from build123d import *

# Parameters (mm, degrees)
SKETCH1_W            = 61
SKETCH1_H            = 90
BOSS_EXTRUDE1_DEPTH  = 8
SKETCH4_W            = 57
SKETCH4_H            = 86
CUT_EXTRUDE1_DEPTH   = 6
SKETCH5_R            = 1.5
BOSS_EXTRUDE12_DEPTH = 2
CUT_EXTRUDE2_REACH   = 79.614
SKETCH6_R            = 3.5
SKETCH6_W            = 17
SKETCH6_H            = 6.5
SKETCH6_W_2          = 9.5
SKETCH6_H_2          = 4
CUT_EXTRUDE3_REACH   = 98.629
SKETCH8_W            = 17.9
SKETCH8_H            = 15.5
SKETCH8_W_2          = 15.1
SKETCH8_H_2          = 16


with BuildPart() as part:
    # Sketch1 → Boss-Extrude1 (new body)
    with BuildSketch(Plane(origin=(0, 0, 0), x_dir=(1, 0, 0), z_dir=(0, 1, 0))):
        Rectangle(SKETCH1_W, SKETCH1_H)
    extrude(amount=BOSS_EXTRUDE1_DEPTH)

    # Sketch4 → Cut-Extrude1 (cut)
    with BuildSketch(Plane(origin=(0, 2, 0), x_dir=(1, 0, 0), z_dir=(0, 1, 0))):
        Rectangle(SKETCH4_W, SKETCH4_H)
    extrude(amount=CUT_EXTRUDE1_DEPTH, mode=Mode.SUBTRACT)

    # Sketch5 → Boss-Extrude12 (add)
    # profile 1 of 4: a face of its own
    with BuildSketch(Plane(origin=(0, 2, 0), x_dir=(1, 0, 0), z_dir=(0, 1, 0))):
        with BuildLine():
            Line((25, -15), (28.5, -15))
            Line((28.5, -15), (28.5, -22))
            Line((28.5, -22), (25, -22))
            ThreePointArc((25, -22), (21.5, -18.5), (25, -15))
        make_face()
        with Locations(Location((25, -18.5, 0), (0, 0, 270))):
            Circle(SKETCH5_R, mode=Mode.SUBTRACT)
    # profile 2 of 4: a face of its own
    with BuildSketch(Plane(origin=(0, 2, 0), x_dir=(1, 0, 0), z_dir=(0, 1, 0))):
        with BuildLine():
            Line((31.5, 39.5), (31.5, 46))
            Line((31.5, 46), (25, 46))
            ThreePointArc((25, 46), (20.403805922, 34.903805922), (31.5, 39.5))
        make_face()
        with Locations(Location((25, 39.5, 0), (0, 0, 270))):
            Circle(SKETCH5_R, mode=Mode.SUBTRACT)
    # profile 3 of 4: a face of its own
    with BuildSketch(Plane(origin=(0, 2, 0), x_dir=(1, 0, 0), z_dir=(0, 1, 0))):
        with BuildLine():
            Line((-20.5, 39.5), (-20.5, 43))
            Line((-20.5, 43), (-28.5, 43))
            Line((-28.5, 43), (-28.5, 36))
            Line((-28.5, 36), (-24, 36))
            ThreePointArc((-24, 36), (-21.525126266, 37.025126266), (-20.5, 39.5))
        make_face()
        with Locations(Location((-24, 39.5, 0), (0, 0, 90))):
            Circle(SKETCH5_R, mode=Mode.SUBTRACT)
    # profile 4 of 4: a face of its own
    with BuildSketch(Plane(origin=(0, 2, 0), x_dir=(1, 0, 0), z_dir=(0, 1, 0))):
        with BuildLine():
            Line((-24, -15), (-28.506473373, -15))
            Line((-28.506473373, -15), (-28.5, -22))
            Line((-28.5, -22), (-24, -22))
            ThreePointArc((-24, -22), (-20.5, -18.5), (-24, -15))
        make_face()
        with Locations(Location((-24, -18.5, 0), (0, 0, 270))):
            Circle(SKETCH5_R, mode=Mode.SUBTRACT)
    extrude(amount=BOSS_EXTRUDE12_DEPTH)

    # Sketch6 → Cut-Extrude2 (cut, up to next)
    with BuildSketch(Plane.ZY.offset(30.5), mode=Mode.PRIVATE) as cut_extrude2_sk1:
        with Locations((10.5, 8.4)):
            Circle(SKETCH6_R)
    cut_extrude2_tool1 = extrude(cut_extrude2_sk1.sketch, amount=-CUT_EXTRUDE2_REACH, mode=Mode.PRIVATE) & part.part
    # Sketch6 → Cut-Extrude2 (cut, up to next)
    with BuildSketch(Plane.ZY.offset(30.5), mode=Mode.PRIVATE) as cut_extrude2_sk2:
        with Locations((-11, 8.15)):
            Rectangle(SKETCH6_W, SKETCH6_H)
    cut_extrude2_tool2 = extrude(cut_extrude2_sk2.sketch, amount=-CUT_EXTRUDE2_REACH, mode=Mode.PRIVATE) & part.part
    # Sketch6 → Cut-Extrude2 (cut, up to next)
    with BuildSketch(Plane.ZY.offset(30.5), mode=Mode.PRIVATE) as cut_extrude2_sk3:
        with Locations((-32.4, 6.9)):
            Rectangle(SKETCH6_W_2, SKETCH6_H_2)
    cut_extrude2_tool3 = extrude(cut_extrude2_sk3.sketch, amount=-CUT_EXTRUDE2_REACH, mode=Mode.PRIVATE) & part.part
    add(cut_extrude2_tool1.solids().sort_by_distance((-30.5, 8.4, 10.5))[0], mode=Mode.SUBTRACT)
    add(cut_extrude2_tool2.solids().sort_by_distance((-30.5, 8.15, -11))[0], mode=Mode.SUBTRACT)
    add(cut_extrude2_tool3.solids().sort_by_distance((-30.5, 6.9, -32.4))[0], mode=Mode.SUBTRACT)

    # Sketch8 → Cut-Extrude3 (cut, up to next)
    with BuildSketch(Plane.XY.offset(45), mode=Mode.PRIVATE) as cut_extrude3_sk1:
        with Locations((-17.25, 12.65)):
            Rectangle(SKETCH8_W, SKETCH8_H)
    cut_extrude3_tool1 = extrude(cut_extrude3_sk1.sketch, amount=-CUT_EXTRUDE3_REACH, mode=Mode.PRIVATE) & part.part
    # Sketch8 → Cut-Extrude3 (cut, up to next)
    with BuildSketch(Plane.XY.offset(45), mode=Mode.PRIVATE) as cut_extrude3_sk2:
        with Locations((1.5, 12.9)):
            Rectangle(SKETCH8_W_2, SKETCH8_H_2)
    cut_extrude3_tool2 = extrude(cut_extrude3_sk2.sketch, amount=-CUT_EXTRUDE3_REACH, mode=Mode.PRIVATE) & part.part
    # Sketch8 → Cut-Extrude3 (cut, up to next)
    with BuildSketch(Plane.XY.offset(45), mode=Mode.PRIVATE) as cut_extrude3_sk3:
        with Locations((19.5, 12.9)):
            Rectangle(SKETCH8_W_2, SKETCH8_H_2)
    cut_extrude3_tool3 = extrude(cut_extrude3_sk3.sketch, amount=-CUT_EXTRUDE3_REACH, mode=Mode.PRIVATE) & part.part
    add(cut_extrude3_tool1.solids().sort_by_distance((-17.25, 12.65, 45))[0], mode=Mode.SUBTRACT)
    add(cut_extrude3_tool2.solids().sort_by_distance((1.5, 12.9, 45))[0], mode=Mode.SUBTRACT)
    add(cut_extrude3_tool3.solids().sort_by_distance((19.5, 12.9, 45))[0], mode=Mode.SUBTRACT)


solid = part.part
For this review, take the finished solid that the model builds, in its own axes (mm). A direction names the side the tool comes from. Round coordinates to 2 decimals unless told otherwise and drop trailing zeros. Order: outer loops, then holes, each group sorted by start corner. A loop starts at its lowest first (then second) coordinate and runs counter-clockwise, first axis right, second up. Notation, with made-up numbers: (-21.75, 78.5) -> (26.25, 78.5) arc R19 ccw to (26.25, 111.5) -> close; hole circle Ø5 at (89, 70.5). An arc over 180 degrees is marked (long way). Write item = value, one per line. Start each with the question number.
1) Take a section at B-B on z = 2.5. State the section outline as (x, y) points.
2) Take a section at C-C on z = 18.5. State the section outline as (x, y) points, plus the area to 3 significant figures.
3) Take a section at A-A on x = 17. State the section outline as (y, z) points.
4) Insertion check: pin 1 (4 mm diameter, centred on y = 4, z = 22.5, fed in from +X); pin 2 (5.5 mm diameter, centred on x = -23.5, z = -38.5, fed in from +Y); pin 3 (5 mm diameter, centred on x = -16, z = -5, fed in from +Y). Each pin has a flat end and moves straight along its axis. Give the tip position at first contact, or say it passes through.
5) Tool access review of faces 5 (the face through (-30.5, 3, 1)), 6 (the face through (27.05, 6, 44)), 7 (the face through (-25.01, 2.99, -38.39)), 8 (the face through (-30, 6, -19.5)): name each direction out of +Z, -Z, +X, -X, +Y, -Y from which nothing blocks a thin tool from reaching the whole face with its end or side.
6) The part is to be moulded in two halves that separate along X. For faces 1 (the face through (0, 2, -1)), 2 (the face through (31, 4, -43)), 3 (the face through (31.5, 3, -43)), 4 (the face through (21.5, 3, 18.6)), say which applies: +X half, -X half, draft (parallel to the pull), parting line (faces both ways), or undercut.
7) To check wall thickness, follow line 1 (X direction, y = 3.6, z = -39.5); line 2 (X direction, y = 3, z = 18.5); line 3 (Y direction, x = 18, z = 13). State the ranges of each line that lie inside material, in increasing order. Write a range as from..to.
Verdict:
q1.outline = (-30.5, 0) -> (30.5, 0) -> (30.5, 8) -> (28.5, 8) -> (28.5, 2) -> (-28.5, 2) -> (-28.5, 8) -> (-30.5, 8) -> close
q2.outline = (-30.5, 0) -> (30.5, 0) -> (30.5, 8) -> (28.5, 8) -> (28.5, 4) -> (26.5, 4) -> (26.5, 2) -> (23.5, 2) -> (23.5, 4) -> (21.5, 4) -> (21.5, 2) -> (-20.5, 2) -> (-20.5, 4) -> (-22.5, 4) -> (-22.5, 2) -> (-25.5, 2) -> (-25.5, 4) -> (-28.5, 4) -> (-28.5, 8) -> (-30.5, 8) -> close
q2.area = 164 mm2
q3.outline = (0, -45) -> (8, -45) -> (8, -43) -> (2, -43) -> (2, 43) -> (4.9, 43) -> (4.9, 45) -> (0, 45) -> close
q4.pin_1 = 30.5
q4.pin_2 = 4
q4.pin_3 = 2
q5.face_5 = +Z, -Z, -X, +Y, -Y
q5.face_6 = +Z, +Y
q5.face_7 = +Y
q5.face_8 = -X, +Y
q6.face_1 = undercut
q6.face_2 = draft
q6.face_3 = +X half
q6.face_4 = undercut
q7.line_1 = -30.5..-25.5, -22.5..-20.5, 18.5..23.5, 26.5..31.5
q7.line_2 = -30.5..-25.5, -22.5..-20.5, 21.5..23.5, 26.5..30.5
q7.line_3 = 0..2
